Verification items for the finished model (mm, model axes). Round coordinates to 2 decimals unless told otherwise and drop trailing zeros. Write each loop counter-clockwise with the first axis right and the second up, starting at its lowest first coordinate (ties: lowest second). Pieces come first, ordered by that corner, then holes. Notation, with made-up numbers: M 71.5,-39 L 79.5,-39 A6 ccw 79.5,-30 Z; hole C 33,20.5 d4. An arc over 180 degrees is marked long. One line per question, with ' | ' between items.
from build123d import *

# Parameters (mm, degrees)
F0_R     = 9.017
F1_DEPTH = 57.15
F2_R     = 4.318
F3_DEPTH = 6.35
F5_R     = 9.017
F7_R     = 5.08


# Not quite as in the source:
# - a fillet or chamfer that OpenCascade refuses, or shapes differently, is made with other operations: its cross-section is extruded or revolved along the edge and cut away or added


with BuildPart() as f1:
    # F0 (on Right) → F1 (new body)
    with BuildSketch(Plane.YZ):
        Circle(F0_R)
    extrude(amount=F1_DEPTH)

    # F2 (on face) → F3 (join)
    with BuildSketch(Plane(origin=(0, 0, 0), x_dir=(0, -1, 0), z_dir=(-1, 0, 0))):
        Circle(F2_R)
    extrude(amount=F3_DEPTH)

    # F5
    f5_edges = [f1.edges().sort_by_distance(p)[0] for p in [
        (57.15, -9.017, 0),
    ]]
    fillet(f5_edges, radius=F5_R)

    # F6: fillet of radius 5.08 on 3 edges, made by hand

    # F6_s1 → F6_t2 (revolve, cut)
    with BuildSketch(Plane.XY):
        with BuildLine():
            ThreePointArc((5.0656923515, 9.017), (1.6109188423, 7.6613710878), (0, 4.318))
            Line((0, 4.318), (0, 9.017))
            Line((0, 9.017), (5.0656923515, 9.017))
        make_face()
    revolve(axis=Axis((0, 0, 0), (1, 0, 0)), mode=Mode.SUBTRACT)

    # F7
    f7_edges = [f1.edges().sort_by_distance(p)[0] for p in [
        (0, 0, 4.318),
        (0, 0, -4.318),
    ]]
    fillet(f7_edges, radius=F7_R)


solid = f1.part
1. Mould release check, pull along Y, two halves, no side actions. Record for faces 1 (the face through (-6.35, 0, 0)), 2 (the face through (-4.9, -1.99, -3.83)): pulls with the +Y half, pulls with the -Y half, needs draft (parallel to the pull), parting line crosses it, or undercut.
Results:
face 1: needs draft | face 2: parting line crosses it
2. Go/stop test with flat-tipped pins: P1, Ø1, axis at y = -1, z = 0, coming from the +X side; P2, Ø1, axis at x = 42, z = 6, coming from the -Y side; P3, Ø3, axis at x = 49, z = 1.5, coming from the -Y side. Record where each tip stops, or that it passes through.
Results:
P1: stops at x = 57.14 | P2: stops at y = -7.15 | P3: stops at y = -9.01
3. Thickness scan on line 1 (Y direction, x = 54.5, z = -0.75); line 2 (X direction, y = -3.5, z = 3.5); line 3 (X direction, y = 6, z = 1.75). Record the ranges inside material, lowest first.
Results:
line 1: y = -6.34 to 6.34 | line 2: x = -1.05 to 55.67 | line 3: x = 0.49 to 54.63
4. Section check B-B, the plane x = 51.5. Record the cut outline in (y, z).
Results:
outline: C 0,0 d16.73
5. Section check A-A, the plane x = 31.5. Record the cut outline in (y, z).
Results:
outline: C 0,0 d18.03
